Geometry: final body of the model. Coordinates: model frame, mm. A direction names the side the tool comes from. Coordinates: 2 decimals unless noted, no trailing zeros. Write each loop counter-clockwise with the first axis right and the second up, starting at its lowest first coordinate (ties: lowest second). Pieces come first, ordered by that corner, then holes. Notation, with made-up numbers: (11.25, -14.5) - (53.25, -14.5) arc R14 cw to (53.25, 9.5) - close; hole circle Ø2 at (3.5, -24.5). An arc over 180 degrees is marked (long way). Put each result on its own line as item: value.
```python
from build123d import *

# Parameters (mm, degrees)
SKETCH1_R           = 4
BOSS_EXTRUDE1_DEPTH = 6
SKETCH2_R           = 2
BOSS_EXTRUDE2_DEPTH = 6
BOSS_EXTRUDE3_DEPTH = 6


with BuildPart() as part:
    # Sketch1 → Boss-Extrude1 (new body)
    with BuildSketch(Plane(origin=(0, 0, 0), x_dir=(1, 0, 0), z_dir=(0, 1, 0))):
        with Locations(Location((0, 0, 0), (0, 0, 270))):
            Circle(SKETCH1_R)
    extrude(amount=BOSS_EXTRUDE1_DEPTH)

    # Sketch2 → Boss-Extrude2 (add)
    with BuildSketch(Plane(origin=(0, 6, 0), x_dir=(1, 0, 0), z_dir=(0, 1, 0))):
        with Locations(Location((0, 0, 0), (0, 0, 270))):
            Circle(SKETCH2_R)
    extrude(amount=BOSS_EXTRUDE2_DEPTH)

    # Sketch3 → Boss-Extrude3 (add)
    with BuildSketch(Plane(origin=(0, 6, 0), x_dir=(1, 0, 0), z_dir=(0, 1, 0))):
        with BuildLine():
            Line((-0.500000000000001, 3.968626966596886), (-0.5, 0.28867513459480454))
            Line((-0.5, 0.28867513459480454), (-3.6869317712168805, -1.551300781406223))
            ThreePointArc((-3.6869317712168805, -1.551300781406223), (-3.4641016151377557, -1.9999999999999982), (-3.186931771216881, -2.4173261851906616))
            Line((-3.186931771216881, -2.4173261851906616), (2.344e-14, -0.5773502691896194))
            Line((2.344e-14, -0.5773502691896194), (3.186931771216881, -2.4173261851906616))
            ThreePointArc((3.186931771216881, -2.4173261851906616), (3.4641016151377553, -1.9999999999999991), (3.6869317712168805, -1.551300781406223))
            Line((3.6869317712168805, -1.551300781406223), (0.5000000000000009, 0.28867513459480254))
            Line((0.5000000000000009, 0.28867513459480254), (0.49999999999999895, 3.968626966596886))
            ThreePointArc((0.49999999999999895, 3.968626966596886), (-1.53e-15, 4), (-0.500000000000001, 3.968626966596886))
        make_face()
    extrude(amount=BOSS_EXTRUDE3_DEPTH)


solid = part.part
```
1. Ray query, probe 1 along Y at (x, z) = (-0.5, 3.5); probe 2 along X at (y, z) = (7, -2.5); probe 3 along Z at (x, y) = (-2.75, 7.25). Return the intervals inside material, ascending. Write a range as from..to.
Answer below:
probe 1: y = 0..6
probe 2: x = -0.5..0.5
probe 3: z = 1.01..2.17
2. Set-up query: faces 4 (the flat face through (2.29, 8.96, 1.9)), 5 (the cylindrical face through (-3.905, 4.583, -0.867)), 6 (the flat face through (0.5, 9, -3)), 7 (the flat face through (0, 0, 0)), 8 (the flat face through (-0.5, 9, -3)). Return all of +Z, -Z, +X, -X, +Y, -Y with unobstructed straight access to the full face (end or side cutting, diameter ignored); none if empty.
Answer below:
face 4: +Z, +Y
face 5: +Y, -Y
face 6: -Z, +X, +Y
face 7: +Z, -Z, +X, -X, -Y
face 8: -Z, -X, +Y
3. Section query D-D (z = -1.75). Return loops of the section in (x, y).
Answer below:
outline: (-3.6, 0) - (3.6, 0) - (3.6, 6) - (0.97, 6) - (0.97, 12) - (-0.97, 12) - (-0.97, 6) - (-3.6, 6) - close
4. Section query B-B (z = 0). Return loops of the section in (x, y), then the cut area to 3 significant figures.
Answer below:
outline: (-4, 0) - (4, 0) - (4, 6) - (2, 6) - (2, 12) - (-2, 12) - (-2, 6) - (-4, 6) - close
area: 72.0 mm²
5. Pin query (flat end, axial travel): pin 1 Ø1 at (y, z) = (9.5, 1.5) entering from -X; pin 2 Ø2 at (y, z) = (5.5, 2.5) entering from +X; pin 3 Ø0.6 at (y, z) = (9, -3.5) entering from +X. Return the tip coordinate at first contact, or that it passes through.
Answer below:
pin 1: stops at x = -3.69
pin 2: stops at x = 3.71
pin 3: stops at x = 0.5
6. Section query C-C (x = 0). Return loops of the section in (y, z), then the cut area to 3 significant figures.
Answer below:
outline: (0, -4) - (12, -4) - (12, 2) - (6, 2) - (6, 4) - (0, 4) - close
area: 84.0 mm²
7. Mould query, pull axis Z, two halves, no side actions, for faces 1 (the flat face through (-2.319, 8.958, 1.916)), 2 (the cylindrical face through (1.743, 8.958, -0.981)), 3 (the flat face through (0, 6, 3)). Classes: +Z half, -Z half, draft (parallel to the pull), parting line (faces both ways), or undercut.
Answer below:
face 1: +Z half
face 2: undercut
face 3: draft
8. Section query A-A (y = 11.25). Return loops of the section in (x, z).
Answer below:
outline: (-3.69, 1.55) - (-1.93, 0.54) arc R2 ccw to (-0.5, -1.94) - (-0.5, -3.97) arc R4 ccw to (0.5, -3.97) - (0.5, -1.94) arc R2 ccw to (1.93, 0.54) - (3.69, 1.55) arc R4 ccw to (3.19, 2.42) - (1.43, 1.4) arc R2 ccw to (-1.43, 1.4) - (-3.19, 2.42) arc R4 ccw to start
